Autodesk Inventor part; units mm, degrees
ref_plane "YZ Plane" through (0, 0, 0) normal (1, 0, 0) x (0, 1, 0)
ref_plane "XZ Plane" through (0, 0, 0) normal (0, 1, 0) x (-1, 0, 0)
ref_plane "XY Plane" through (0, 0, 0) normal (0, 0, 1) x (1, 0, 0)
sketch "Sketch1" plane through (0, 0, 0) normal (0, 0, 1) x (1, 0, 0)
  line L0 (0, 0) -> (0, 100)
  line L1 (0, 100) -> (120, 100)
  line L2 (120, 100) -> (120, 0)
  line L3 (120, 0) -> (0, 0)
  circle A0 centre (60, 50) radius 25
  line L4 (0, 0) -> (0, 6)
  line L5 (0, 6) -> (10, 6)
  line L6 (10, 6) -> (10, 0)
  line L7 (10, 0) -> (30, 0)
  line L8 (30, 0) -> (30, 6)
  line L9 (30, 6) -> (50, 6)
  line L10 (50, 6) -> (50, 0)
  line L11 (50, 0) -> (70, 0)
  line L12 (70, 0) -> (70, 6)
  line L13 (70, 6) -> (90, 6)
  line L14 (90, 6) -> (90, 0)
  line L15 (90, 0) -> (110, 0)
  line L16 (110, 0) -> (110, 6)
  line L17 (110, 6) -> (120, 6)
  dimension "d3" = 100
  dimension "d4" = 120
  dimension "d6" = 50
  dimension "d9" = 50
  dimension "d10" = 60
  dimension "d11" = 6
  dimension "d12" = 10
  dimension "d13" = 20
  dimension "d14" = 20
  dimension "d15" = 20
  dimension "d16" = 20
  dimension "d17" = 20
extrude "Extrusion1" add sketch "Sketch1" against normal blind 5 contours L0 L1 L2 L17 L16 L3 L14 L13 L12 L10 L9 L8 L6 L5
properties part number "Archimedes Screw Border1"
For this review, take the finished solid that the model builds, in its own axes (mm). A direction names the side the tool comes from. Coordinates: 2 decimals unless noted, no trailing zeros. Write each loop counter-clockwise with the first axis right and the second up, starting at its lowest first coordinate (ties: lowest second). Pieces come first, ordered by that corner, then holes. Notation, with made-up numbers: (-1.5, 72.5) - (9.5, 72.5) arc R27 ccw to (9.5, 109.5) - close; hole circle Ø5 at (66, 53.25). An arc over 180 degrees is marked (long way). Put each result on its own line as item: value.
1. Mouldability with a two-part tool opening along X and no side actions: class faces 1 (the cylindrical face through (40, 35, -2)), 2 (the flat face through (46, 73, -5)), 3 (the flat face through (110, 3, -2)) as released by +X, released by -X, zero draft, split by the parting line, or undercut.
Values found:
face 1: undercut
face 2: zero draft
face 3: released by +X
2. Add section A-A, the plane x = 60. Give the boundary of the cut face in (y, z), then the cut area to 3 significant figures.
Values found:
outline: (0, -5) - (25, -5) - (25, 0) - (0, 0) - close; (75, -5) - (100, -5) - (100, 0) - (75, 0) - close
area: 250 mm²
3. Wall thickness on probe 1 along Y at (x, z) = (60, -2.6); probe 2 along X at (y, z) = (72.5, -3.8); probe 3 along X at (y, z) = (29, -2): over which ranges is each line inside the solid? List them lowest first.
Values found:
probe 1: 0 to 25, 75 to 100
probe 2: 0 to 49.1, 70.9 to 120
probe 3: 0 to 46.44, 73.56 to 120
4. Add section B-B, the plane z = -1.25. Give the boundary of the cut face in (x, y), then the cut area to 3 significant figures.
Values found:
outline: (0, 6) - (10, 6) - (10, 0) - (30, 0) - (30, 6) - (50, 6) - (50, 0) - (70, 0) - (70, 6) - (90, 6) - (90, 0) - (110, 0) - (110, 6) - (120, 6) - (120, 100) - (0, 100) - close; hole circle Ø50 at (60, 50)
area: 9,680 mm²
5. Machinability: for faces 4 (the flat face through (59, 100, -2)), 5 (the flat face through (5, 6, -2)), 6 (the flat face through (90, 3, -2)), which of the approach directions +Z, -Z, +X, -X, +Y, -Y give a long, thin tool a straight path to every point of the face, cutting with its end or side? Answer none if there is none.
Values found:
face 4: +Z, -Z, +X, -X, +Y
face 5: +Z, -Z, -X, -Y
face 6: +Z, -Z, -Y
6. For pin 1 (1.5 mm diameter, centred on x = 75.5, z = -1.5, fed in from -Y); pin 2 (1.5 mm diameter, centred on y = 3, z = -3.5, fed in from +X); pin 3 (2.5 mm diameter, centred on y = 3, z = -3, fed in from -X), all flat-tipped, find the tip position at first contact; note any pin that passes through.
Values found:
pin 1: y = 6
pin 2: x = 110
pin 3: x = 10
7. Add section C-C, the plane y = 50. Give the boundary of the cut face in (x, z).
Values found:
outline: (0, -5) - (35, -5) - (35, 0) - (0, 0) - close; (85, -5) - (120, -5) - (120, 0) - (85, 0) - close
